from build123d import *

# Parameters (mm, degrees)
F1_DEPTH = 50.8
F2_R     = 4.7625
F3_DEPTH = 12.7
F5_DEPTH = 3.175


with BuildPart() as f1:
    # F0 (on Front) → F1 (new body)
    with BuildSketch(Plane.XZ):
        Polygon((38.1, -15.875), (38.1, -3.175), (-25.4, -3.175), (-25.4, -15.875), (-12.7, -15.875), (-12.7, -22.225), (-12.7, -42.06454), (25.4, -42.06454), (25.4, -22.225), (25.4, -15.875), align=None)
    extrude(amount=F1_DEPTH)

    # F2 (on face) → F3 (cut)
    with BuildSketch(Plane.YZ.offset(38.1)):
        with Locations((-25.4, -9.525)):
            Circle(F2_R)
    extrude(amount=-F3_DEPTH, mode=Mode.SUBTRACT)

    # F4 (on face) → F5 (cut)
    with BuildSketch(Plane.YZ.offset(38.1)):
        with BuildLine():
            Line((-38.1, -14.2875), (-25.4, -14.2875))
            Line((-25.4, -14.2875), (-12.7, -14.2875))
            ThreePointArc((-12.7, -14.2875), (-11.801974, -13.915526), (-11.43, -13.0175))
            Line((-11.43, -13.0175), (-11.43, -9.8425))
            Line((-11.43, -9.8425), (-11.43, -6.0325))
            ThreePointArc((-11.43, -6.0325), (-11.801974, -5.134474), (-12.7, -4.7625))
            Line((-12.7, -4.7625), (-18.372404, -4.7625))
            Line((-18.372404, -4.7625), (-25.4, -4.7625))
            Line((-25.4, -4.7625), (-38.1, -4.7625))
            ThreePointArc((-38.1, -4.7625), (-38.998026, -5.134474), (-39.37, -6.0325))
            Line((-39.37, -6.0325), (-39.37, -13.0175))
            ThreePointArc((-39.37, -13.0175), (-38.998026, -13.915526), (-38.1, -14.2875))
        make_face()
    extrude(amount=-F5_DEPTH, mode=Mode.SUBTRACT)


solid = f1.part
Can you work these out from the model? Positions are in its coordinate system, mm. A direction names the side the tool comes from. Give positions to 0.01 mm unless a question says otherwise; leave off trailing zeros. Loops run counter-clockwise (first coordinate to the right, second up) from the corner with the lowest first, then second, coordinate; pieces in that order, holes last. Notation, with made-up numbers: (71, 50) -> (95, 50) arc R27 ccw to (95, 86) -> close; hole circle Ø7 at (82, 37). An arc over 180 degrees is marked (long way). Return JSON: item names as keys, results as strings.
Q1. I want a section at A-A, the plane y = -43. List the corners of the cut face in (x, z) for me (3 decimals).
Checks:
{"outline": "(-25.4, -15.875) -> (-12.7, -15.875) -> (-12.7, -42.065) -> (25.4, -42.065) -> (25.4, -15.875) -> (38.1, -15.875) -> (38.1, -3.175) -> (-25.4, -3.175) -> close"}
Q2. We'd pull the mould along Y, two halves only. Please class faces 1 (the face through (25.4, -25, -29)), 2 (the face through (6, 0, -18)), 3 (the face through (37, -11.43, -10)): released by +Y, released by -Y, zero draft, split by the parting line, or undercut.
Checks:
{"face 1": "zero draft", "face 2": "released by +Y", "face 3": "undercut"}
Q3. I need wall thicknesses on probe 1 along Z at (x, y) = (30, -25.4) (1 decimal); probe 2 along X at (y, z) = (-48.5, -18); probe 3 along X at (y, z) = (-31.5, -13.5) (3 decimals). Which ranges of each line are inside material? Lowest first, please.
Checks:
{"probe 1": "z = -15.9 to -14.3, -4.8 to -3.2", "probe 2": "x = -12.7 to 25.4", "probe 3": "x = -25.4 to 34.925"}
Q4. On a 3-axis mill with a long thin cutter (end or side, diameter ignored), from which of +Z, -Z, +X, -X, +Y, -Y can I reach the whole of each face in a straight line? I mean faces 4 (the face through (-19, -25, -15.875)), 5 (the face through (32, -25, -15.875)), 6 (the face through (37, -26, -14.288)), 7 (the face through (-25.4, -25, -9)). Say none if no direction works.
Checks:
{"face 4": "-Z, -X, +Y, -Y", "face 5": "-Z, +X, +Y, -Y", "face 6": "+X", "face 7": "+Z, -Z, -X, +Y, -Y"}
Q5. For pin 1 Ø3 at (y, z) = (-35.5, -8) entering from +X (3 decimals); pin 2 Ø8 at (y, z) = (-37, -28.5) entering from +X; pin 3 Ø10 at (x, y) = (33, -24) entering from -Z (3 decimals), each with a flat end and sliding along its axis, tell me the tip position at first contact or that it passes through.
Checks:
{"pin 1": "stops at x = 34.925", "pin 2": "stops at x = 25.4", "pin 3": "stops at z = -15.875"}
Q6. I want a section at B-B, the plane z = -18. List the corners of the cut face in (x, y) for me, then the cut area to 3 significant figures.
Checks:
{"outline": "(-12.7, -50.8) -> (25.4, -50.8) -> (25.4, 0) -> (-12.7, 0) -> close", "area": "1,940 mm2"}
Q7. I want a section at C-C, the plane y = -19. List the corners of the cut face in (x, z) for me (1 decimal).
Checks:
{"outline": "(-25.4, -15.9) -> (-12.7, -15.9) -> (-12.7, -42.1) -> (25.4, -42.1) -> (25.4, -15.9) -> (38.1, -15.9) -> (38.1, -14.3) -> (34.9, -14.3) -> (34.9, -4.8) -> (38.1, -4.8) -> (38.1, -3.2) -> (-25.4, -3.2) -> close"}
